Input: part model. Units: mm. Frame: model coordinates. A direction names the side the tool comes from. Give positions to 0.01 mm unless a question says otherwise; leave off trailing zeros. Loops run counter-clockwise (first coordinate to the right, second up) from the corner with the lowest first, then second, coordinate; pieces in that order, holes last. Notation, with made-up numbers: (-18, -26) - (2, -26) arc R24 cw to (2, 10) - close; hole circle Ø9 at (-9, -34.75). An arc over 180 degrees is marked (long way). One line per item, written item: value.
Autodesk Inventor part; units mm, degrees
ref_plane "YZ Plane" through (0, 0, 0) normal (1, 0, 0) x (0, 1, 0)
ref_plane "XZ Plane" through (0, 0, 0) normal (0, 1, 0) x (-1, 0, 0)
ref_plane "XY Plane" through (0, 0, 0) normal (0, 0, 1) x (1, 0, 0)
sketch "Sketch1" plane through (0, 0, 0) normal (0, 1, 0) x (-1, 0, 0)
  circle A0 centre (0, 0) radius 360
  circle A1 centre (0, 0) radius 335 construction
  circle A2 centre (335, 0) radius 7.1437
  circle A3 centre (0, 0) radius 50.8
  circle A4 centre (220, 0) radius 50.8
  circle A5 centre (-220, 0) radius 50.8
  circle A6 centre (0, -190) radius 25.4
  circle A7 centre (0, 190) radius 25.4
  circle A8 centre (0, 0) radius 190 construction
  circle A9 centre (0, 0) radius 220 construction
  dimension "d1" = 670
  dimension "d0" = 720
  dimension "d2" = 14.2875
  dimension "d3" = 101.6
  dimension "d4" = 101.6
  dimension "d5" = 101.6
  dimension "d6" = 50.8
  dimension "d7" = 50.8
  dimension "d8" = 380
  dimension "d23" = 440
extrude "Extrusion1" add sketch "Sketch1" along normal blind 8 contours A0 | A2
extrude "Extrusion2" cut sketch "Sketch1" along normal through all contours A2
pattern_circular "Circular Pattern1" count 24 over 360 about axis through (0, 0, 0) along (0, 1, 0) of "Extrusion2"
sketch "Sketch2" plane through (0, 8, 0) normal (0, 1, 0) x (1, 0, 0)
  circle A0 centre (-323.5852, 86.7044) radius 7.1437
  circle A1 centre (-290.1185, 167.5) radius 7.1437
  circle A2 centre (-236.8808, 236.8808) radius 7.1437
  circle A3 centre (-167.5, 290.1185) radius 7.1437
  circle A4 centre (-86.7044, 323.5852) radius 7.1437
  circle A5 centre (0, 335) radius 7.1437
  circle A6 centre (86.7044, 323.5852) radius 7.1437
  circle A7 centre (167.5, 290.1185) radius 7.1437
  circle A8 centre (236.8808, 236.8808) radius 7.1437
  circle A9 centre (290.1185, 167.5) radius 7.1437
  circle A10 centre (323.5852, 86.7044) radius 7.1437
  circle A11 centre (335, 0) radius 7.1437
  circle A12 centre (323.5852, -86.7044) radius 7.1437
  circle A13 centre (290.1185, -167.5) radius 7.1437
  circle A14 centre (236.8808, -236.8808) radius 7.1437
  circle A15 centre (167.5, -290.1185) radius 7.1437
  circle A16 centre (86.7044, -323.5852) radius 7.1437
  circle A17 centre (0, -335) radius 7.1437
  circle A18 centre (-86.7044, -323.5852) radius 7.1437
  circle A19 centre (-167.5, -290.1185) radius 7.1437
  circle A20 centre (-236.8808, -236.8808) radius 7.1437
  circle A21 centre (-290.1185, -167.5) radius 7.1437
  circle A22 centre (-323.5852, -86.7044) radius 7.1437
  circle A23 centre (-335, 0) radius 7.1437
  circle A24 centre (0, 0) radius 360
  circle A25 centre (0, 0) radius 50.8
  circle A26 centre (-220, 0) radius 50.8
  circle A27 centre (220, 0) radius 50.8
  circle A28 centre (0, 190) radius 25.4
  circle A29 centre (0, -190) radius 25.4
  circle A30 centre (0, 190) radius 25.4
  circle A31 centre (0, 190) radius 31.4
  circle A32 centre (220, 0) radius 50.8
  circle A33 centre (220, 0) radius 58.8
  circle A34 centre (0, 0) radius 58.8
  circle A35 centre (0, -190) radius 31.4
  circle A36 centre (-220, 0) radius 58.8
  dimension "d16" = 6
  dimension "d17" = 8
  dimension "d18" = 8
  dimension "d19" = 8
  dimension "d20" = 6
extrude "Extrusion3" add sketch "Sketch2" along normal mid plane 45 contours A31 | A33 | A34 | A35 | A36
equation "\"d4\" = d3"
equation "\"d5\" = d3"
equation "\"d6\" = 0.5 * d3"
equation "\"d7\" = 0.5 * d3"
equation "\"d18\" = d17"
equation "\"d19\" = d17"
equation "\"d20\" = d16"
equation "\"Part_Area\" = 88962.969866"
properties part number "Tapa2" material "Steel ASTM A36"
Item 1: Section B-B, the plane z = 200. Output: boundary loops of the cut face in (x, y).
Verdict:
outline: (-299.33, 0) - (-29.77, 0) - (-29.77, -14.5) - (-23.35, -14.5) - (-23.35, 30.5) - (-29.77, 30.5) - (-29.77, 8) - (-299.33, 8) - close; (23.35, -14.5) - (29.77, -14.5) - (29.77, 0) - (299.33, 0) - (299.33, 8) - (29.77, 8) - (29.77, 30.5) - (23.35, 30.5) - close
Item 2: Pin query (flat end, axial travel): P1, Ø23, axis at x = 86.7, z = 323.59, coming from the +Y side; P2, Ø2, axis at y = 7, z = 133.5, coming from the +X side; P3, Ø12, axis at x = 244, z = -57, coming from the -Y side; P4, Ø12, axis at x = -234.5, z = 280, coming from the -Y side. Return the tip coordinate at first contact, or that it passes through.
Verdict:
P1: stops at y = 8
P2: stops at x = 334.73
P3: stops at y = -14.5
P4: stops at y = 0
Item 3: Section A-A, the plane y = -7. Count the separate pieces of the cut face and the enclosed holes in it, and give its area (3 significant figures).
Verdict:
separate pieces: 5
enclosed holes: 5
area: 10,400 mm^2
Item 4: Material intervals for L1, parallel to X at y = 16.5, z = 0; L2, parallel to Z at x = 0, y = -6.5; L3, parallel to Z at x = -174, y = 7 (1 decimal), sorted ascending.
Verdict:
L1: x = -278.8 to -270.8, -169.2 to -161.2, -58.8 to -50.8, 50.8 to 58.8, 161.2 to 169.2, 270.8 to 278.8
L2: z = -221.4 to -215.4, -164.6 to -158.6, -58.8 to -50.8, 50.8 to 58.8, 158.6 to 164.6, 215.4 to 221.4
L3: z = -315.2 to -293.1, -287.2 to -21.6, 21.6 to 287.2, 293.1 to 315.2
Item 5: Access query for faces 5 (the face through (176, -14.5, 26)), 6 (the face through (-278.743, 19.092, 2.585)), 7 (the face through (-6.807, -7.148, -159.347)). Directions: +Z, -Z, +X, -X, +Y, -Y. A direction counts if a zero-diameter tool reaches every point of the face in a straight line with its end or side. Return the directions, or none.
Verdict:
face 5: +Z, -Z, +X, -X, -Y
face 6: +Y
face 7: -Y
Item 6: Section C-C, the plane x = 118. Output: boundary loops of the cut face in (y, z).
Verdict:
outline: (0, -340.11) - (8, -340.11) - (8, 340.11) - (0, 340.11) - close
Item 7: Draft query along Z for faces 1 (the face through (-6.807, 19.092, -220.653)), 2 (the face through (161.257, -7.148, -2.585)), 3 (the face through (-2.47, 30.5, 215.44)), 4 (the face through (-12.75, 19.09, -57.4)). Return one class per face: pulls with the +Z half, pulls with the -Z half, needs draft (parallel to the pull), parting line crosses it, or undercut.
Verdict:
face 1: undercut
face 2: parting line crosses it
face 3: needs draft
face 4: undercut
